from build123d import *

# Parameters (mm, degrees)
PAD001_DEPTH        = 130
POCKET_DEPTH        = 77
SKETCH003_R         = 2.75
HOLE_DEPTH          = 150.001
HOLE001_D           = 5.5
HOLE001_DEPTH       = 25
HOLE001_CBORE_D     = 13
HOLE001_CBORE_DEPTH = 6.4
SKETCH012_W         = 40
SKETCH012_H         = 91.25
PAD004_DEPTH        = 52
POCKET003_DEPTH     = 54
POCKET003_TAPER     = 30
POCKET004_DEPTH     = 36
PAD006_DEPTH        = 52
SKETCH028_R         = 10.65
SKETCH028_R_2       = 13
POCKET009_DEPTH     = 5
POCKET011_DEPTH     = 102


with BuildPart() as part:
    # Sketch001 → Pad001 (new body)
    with BuildSketch(Plane.XY):
        Polygon((300, 70), (0, 70), (-5, 57.5), (-5, 51), (310, 51), (310, 60), align=None)
    extrude(amount=PAD001_DEPTH)

    # Sketch002 → Pocket (cut)
    with BuildSketch(Plane.XZ):
        Polygon((310, 60), (130, 150), (310, 150), align=None)
    extrude(amount=-POCKET_DEPTH, mode=Mode.SUBTRACT)

    # Sketch003 → Hole (cut, through all)
    with BuildSketch(Plane.XY.offset(150)):
        with Locations((100, 60)):
            Circle(SKETCH003_R)
        with Locations((200, 60)):
            Circle(SKETCH003_R)
        with Locations((285, 60)):
            Circle(SKETCH003_R)
        with Locations((25, 60)):
            Circle(SKETCH003_R)
    extrude(amount=-HOLE_DEPTH, mode=Mode.SUBTRACT)

    # Hole001
    with Locations(Plane(origin=(0, 70, 0), x_dir=(1, 0, 0), z_dir=(0, 1, 0))):
        with Locations((20, -20), (70, -20), (120, -20), (170, -20), (220, -20), (270, -20)):
            CounterBoreHole(HOLE001_D / 2, HOLE001_CBORE_D / 2, HOLE001_CBORE_DEPTH, depth=HOLE001_DEPTH)

    # Sketch012 → Pad004 (join)
    with BuildSketch(Plane.XZ):
        with Locations((15, 84.375)):
            Rectangle(SKETCH012_W, SKETCH012_H)
    extrude(amount=-PAD004_DEPTH)

    # Sketch014 → Pocket003 (cut)
    with BuildSketch(Plane.XY.offset(130)):
        Polygon((-50, -40), (-50, 100), (60, 100), align=None)
    extrude(amount=-POCKET003_DEPTH, taper=POCKET003_TAPER, mode=Mode.SUBTRACT)

    # Sketch016 → Pocket004 (cut)
    with BuildSketch(Plane.YZ.offset(35)):
        Polygon((0, 113), (0, 29), (51, 29), (51, 95), (30, 113), align=None)
    extrude(amount=-POCKET004_DEPTH, mode=Mode.SUBTRACT)

    # Sketch018 → Pad006 (join)
    with BuildSketch(Plane.XZ):
        Polygon((290, 70), (290, 39), (310, 39), (310, 60), align=None)
    extrude(amount=-PAD006_DEPTH)

    # Sketch028 → Pocket009 (cut)
    with BuildSketch(Plane.YZ):
        with Locations((20, 95)):
            Circle(SKETCH028_R)
        with Locations((25, 60)):
            Circle(SKETCH028_R_2)
    extrude(amount=-POCKET009_DEPTH, mode=Mode.SUBTRACT)

    # Sketch136 → Pocket011 (cut)
    with BuildSketch(Plane.XZ):
        Polygon((-20, 140), (-20, 105), (30, 140), align=None)
    extrude(amount=-POCKET011_DEPTH, mode=Mode.SUBTRACT)


with BuildPart() as part_1:
    # Body001 placement: moved
    add(part.part.moved(Location((0, 0, 10))))


solid = part_1.part
Input: part model. Units: mm. Frame: model coordinates. A direction names the side the tool comes from. Give positions to 0.01 mm unless a question says otherwise; leave off trailing zeros. Order: outer loops, then holes, each group sorted by start corner. A loop starts at its lowest first (then second) coordinate and runs counter-clockwise, first axis right, second up. Notation, with made-up numbers: (-24, 11) - (32, 11) arc R23 cw to (32, 24) - close; hole circle Ø8 at (40.5, 49). An arc over 180 degrees is marked (long way). Answer as a JSON object with one key per item and string values. Group by question number.
Q1. Cut plane A-A, the plane y = 20. Output: boundary loops of the cut face in (x, z).
Q2. Mould query, pull axis X, two halves, no side actions, for faces 4 (the face through (72.747, 57.212, 29.879)), 5 (the face through (-2.97, 23.31, 82.89)), 6 (the face through (-2.465, 63.838, 52.868)). Classes: pulls with the +X half, pulls with the -X half, needs draft (parallel to the pull), parting line crosses it, or undercut.
Q3. First-contact query: pin 1 Ø10.5 at (y, z) = (18, 120.5) entering from +X; pin 2 Ø1.2 at (x, y) = (-3.5, 30) entering from -Z; pin 3 Ø6.5 at (x, z) = (70, 30) entering from +Y. Flat tips, straight axial feed; report the tip coordinate or a pass-through.
Q4. Cut plane D-D, the plane x = 56.5. Output: boundary loops of the cut face in (y, z), then the cut area to 3 significant figures.
Q5. Line query: probe 1 along Z at (x, y) = (170, 65.5); probe 2 along X at (y, z) = (39.5, 58); probe 3 along Y at (x, z) = (38, 44.5). Output: solid intervals per line, ascending.
Q6. Cut plane C-C, the plane x = 182. Output: boundary loops of the cut face in (y, z).
Q7. Set-up query: faces 1 (the face through (152, 70, 74)), 2 (the face through (123, 63.6, 30)), 3 (the face through (17, 15, 123)). Return all of +Z, -Z, +X, -X, +Y, -Y with unobstructed straight access to the full face (end or side cutting, diameter ignored); none if empty.
Q8. Cut plane B-B, the plane z = 52.5. Output: boundary loops of the cut face in (x, y), then the cut area to 3 significant figures.
Results:
{
 "1": {"outline": "(-5, 48.75) - (-1, 48.75) - (-1, 58) - (-5, 58) - close; (-5, 82) - (-1, 82) - (-1, 94.35) - (-5, 94.35) - close; (-5, 115.65) - (-1, 115.65) - (-1, 123) - (35, 123) - (35, 140) - (15.71, 140) - (-5, 125.5) - close; (290, 49) - (310, 49) - (310, 70) - (290, 80) - close"},
 "2": {"face 4": "undercut", "face 5": "needs draft", "face 6": "pulls with the -X half"},
 "3": {"pin 1": "x = 35", "pin 2": "z = 48.75", "pin 3": "y = 63.6"},
 "4": {"outline": "(51, 10) - (70, 10) - (70, 140) - (51, 140) - close", "area": "2,470 mm^2"},
 "5": {"probe 1": "10 to 23.5, 36.5 to 140", "probe 2": "-5 to -1, 290 to 310", "probe 3": "51 to 70"},
 "6": {"outline": "(51, 10) - (70, 10) - (70, 134) - (51, 134) - close"},
 "7": {"face 1": "+Z, -Z, +X, -X, +Y", "face 2": "+Y", "face 3": "-Z, +X, -Y"},
 "8": {"outline": "(-5, 0) - (-1, 0) - (-1, 51) - (290, 51) - (290, 0) - (310, 0) - (310, 60) - (300, 70) - (0, 70) - (-5, 57.5) - close; hole circle Ø5.5 at (25, 60); hole circle Ø5.5 at (100, 60); hole circle Ø5.5 at (200, 60); hole circle Ø5.5 at (285, 60)", "area": "7,030 mm^2"}
}
